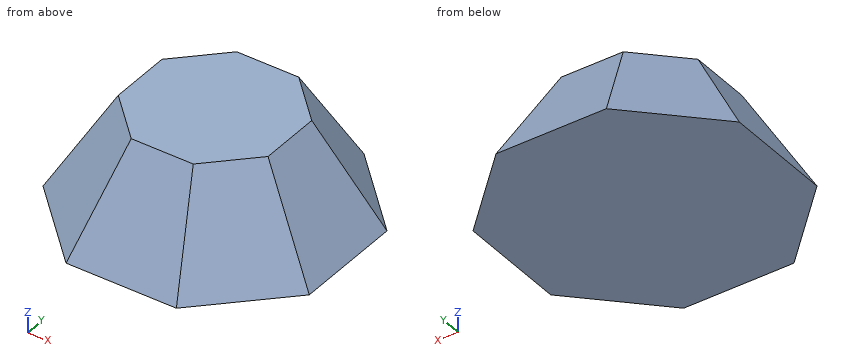
from build123d import *

# Parameters (mm, degrees)
RESSALTO_EXTRUS_O1_DEPTH = 40
RESSALTO_EXTRUS_O1_TAPER = 30


with BuildPart() as part:
    # Esboço1 → Ressalto-extrusão1 (new body)
    with BuildSketch(Plane.XY):
        Polygon((52.78, -21.862191822), (52.78, 21.862191822), (21.862191822, 52.78), (-21.862191822, 52.78), (-52.78, 21.862191822), (-52.78, -21.862191822), (-21.862191822, -52.78), (21.862191822, -52.78), align=None)
    extrude(amount=RESSALTO_EXTRUS_O1_DEPTH, taper=RESSALTO_EXTRUS_O1_TAPER)


solid = part.part
The model under review builds one solid part; all positions refer to its coordinate system, in mm. Give positions to 0.01 mm unless a question says otherwise; leave off trailing zeros. Order: outer loops, then holes, each group sorted by start corner. A loop starts at its lowest first (then second) coordinate and runs counter-clockwise, first axis right, second up. Notation, with made-up numbers: (6.25, 3) -> (42.25, 3) arc R28 cw to (42.25, 32) -> close; hole circle Ø8 at (-21.75, 70). An arc over 180 degrees is marked (long way). Write item = value, one per line. Start each with the question number.
(1) Take a section at B-B (x = -15.5). Write out the cut boundary in (y, z), plus the area to 3 significant figures.
(2) Take a section at D-D (z = 35). Write out the cut boundary in (x, y), plus the area to 3 significant figures.
(3) Take a section at C-C (y = 19). Write out the cut boundary in (x, z), plus the area to 3 significant figures.
(4) For pin 1 Ø1 at (x, y) = (38, -15.5) entering from +Z; pin 2 Ø2 at (y, z) = (20.5, 34) entering from +X; pin 3 Ø5 at (x, y) = (30, -4.5) entering from +Z; pin 4 Ø2 at (x, z) = (26.5, 11.5) entering from -Y, all flat-tipped, find the tip position at first contact; note any pin that passes through.
(5) Take a section at A-A (z = 10). Write out the cut boundary in (x, y).
(6) For L1, parallel to X at y = 15.5, z = 32; L2, parallel to Z at x = -35, y = 13; L3, parallel to Y at x = -9, z = 9.5, list the stretches that pass through material, from the lowest coordinate up. Write a range as from..to.
Returned:
q1.outline = (-52.78, 0) -> (52.78, 0) -> (37.42, 26.6) -> (26.48, 40) -> (-26.48, 40) -> (-37.42, 26.6) -> close
q1.area = 3,260 mm²
q2.outline = (-32.57, -13.49) -> (-13.49, -32.57) -> (13.49, -32.57) -> (32.57, -13.49) -> (32.57, 13.49) -> (13.49, 32.57) -> (-13.49, 32.57) -> (-32.57, 13.49) -> close
q2.area = 3,520 mm²
q3.outline = (-52.78, 0) -> (52.78, 0) -> (45.87, 11.97) -> (22.98, 40) -> (-22.98, 40) -> (-45.87, 11.97) -> close
q3.area = 3,110 mm²
q4.pin_1 = 26.47
q4.pin_2 = 27.67
q4.pin_3 = 40
q4.pin_4 = -40.04
q5.outline = (-47.01, -19.47) -> (-19.47, -47.01) -> (19.47, -47.01) -> (47.01, -19.47) -> (47.01, 19.47) -> (19.47, 47.01) -> (-19.47, 47.01) -> (-47.01, 19.47) -> close
q6.L1 = -33.01..33.01
q6.L2 = 0..30.8
q6.L3 = -47.3..47.3
